The drawing under review shows one solid part. Ordinate dimensions are in mm from its lowest x, y, z. Coordinates: 2 decimals unless noted, no trailing zeros. Write each loop counter-clockwise with the first axis right and the second up, starting at its lowest first coordinate (ties: lowest second). Pieces come first, ordered by that corner, then holes.
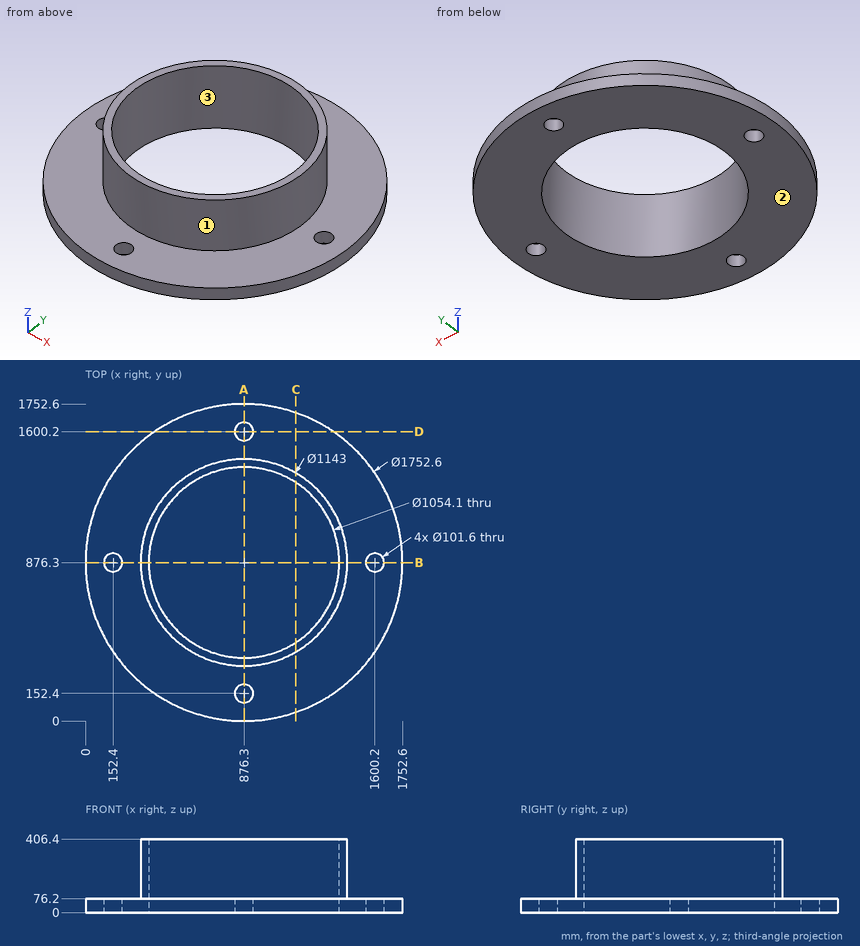
1) The part is to be moulded in two halves that separate along Y. For the marked faces 1, 2 and 3, say which applies: pulls with the +Y half, pulls with the -Y half, needs draft (parallel to the pull), parting line crosses it, or undercut.
2) For L1, parallel to X at y = 876, z = 38; L2, parallel to Z at x = 1364.5, y = 1418, list the stretches that pass through material, from the lowest coordinate up.
3) Consider section A-A (x = 876.3). Give the boundary of the cut face in (y, z), then the cut area to 3 significant figures.
4) Consider section C-C (x = 1163). Give the boundary of the cut face in (y, z).
5) Consider section D-D (y = 1600.2). Give the boundary of the cut face in (x, z).
6) Clearance check with flat-ended pins moving along their axes: P1, Ø6, axis at x = 573, z = 252.5, coming from the +Y side; P2, Ø2, axis at x = 1533, y = 1327.5, coming from the +Z side; P3, Ø3, axis at y = 931, z = 354.5, coming from the +X side. State where each tip first meets the part, or that it passes through.
Results:
1. face 1: parting line crosses it
1. face 2: needs draft
1. face 3: undercut
2. L1: x = 0 to 101.6, 203.2 to 349.25, 1403.35 to 1549.4, 1651 to 1752.6
2. L2: z = 0 to 76.2
3. outline: (0, 0) - (101.6, 0) - (101.6, 76.2) - (0, 76.2) - close; (203.2, 0) - (349.25, 0) - (349.25, 406.4) - (304.8, 406.4) - (304.8, 76.2) - (203.2, 76.2) - close; (1403.35, 0) - (1549.4, 0) - (1549.4, 76.2) - (1447.8, 76.2) - (1447.8, 406.4) - (1403.35, 406.4) - close; (1651, 0) - (1752.6, 0) - (1752.6, 76.2) - (1651, 76.2) - close
3. area: 67,100 mm2
4. outline: (48.23, 0) - (434.05, 0) - (434.05, 406.4) - (381.92, 406.4) - (381.92, 76.2) - (48.23, 76.2) - close; (1318.55, 0) - (1704.37, 0) - (1704.37, 76.2) - (1370.68, 76.2) - (1370.68, 406.4) - (1318.55, 406.4) - close
5. outline: (382.47, 0) - (825.5, 0) - (825.5, 76.2) - (382.47, 76.2) - close; (927.1, 0) - (1370.13, 0) - (1370.13, 76.2) - (927.1, 76.2) - close
6. P1: stops at y = 1362.54
6. P2: stops at z = 76.2
6. P3: stops at x = 1445.32
